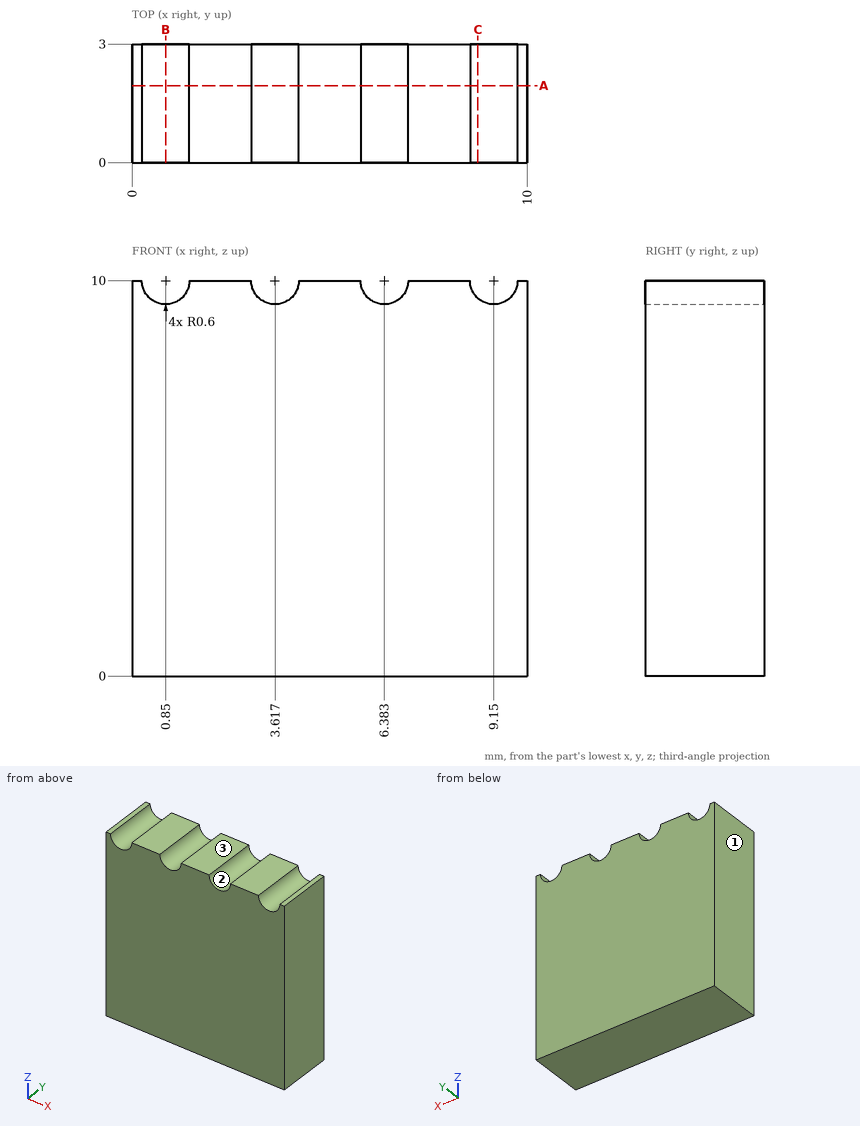
Part print with two shaded views. Sizes in mm from the minimum x, y, z corner. Round coordinates to 2 decimals unless told otherwise and drop trailing zeros. Order: outer loops, then holes, each group sorted by start corner. A loop starts at its lowest first (then second) coordinate and runs counter-clockwise, first axis right, second up. Notation, with made-up numbers: (86, 83) - (137, 83) arc R7 cw to (137, 90) - close; hole circle Ø7 at (22, 86). An arc over 180 degrees is marked (long way). Answer as CSV lines item,"result". Start each with the question number.
1. Saw through at B-B, the plane x = 0.85. Write the cut outline in (y, z).
2. Saw through at A-A, the plane y = 1.95. Write the cut outline in (x, z).
3. Saw through at C-C, the plane x = 8.75. Write the cut outline in (y, z).
4. Drill centre lines: L1, parallel to Z at x = 9.25, y = 1.7; L2, parallel to Z at x = 6, y = 1.6. Where is each one in solid material? Low to high. Write a range as [from, to].
5. Pull direction X, two halves, no side cores. Call the marked faces 1, 2 and 3: +X half, -X half, draft (parallel to the pull), parting line (faces both ways), or undercut.
Model answer:
1,outline,"(0, 0) - (3, 0) - (3, 9.4) - (0, 9.4) - close"
2,outline,"(0, 0) - (10, 0) - (10, 10) - (9.75, 10) arc R0.6 cw to (8.55, 10) - (6.98, 10) arc R0.6 cw to (5.78, 10) - (4.22, 10) arc R0.6 cw to (3.02, 10) - (1.45, 10) arc R0.6 cw to (0.25, 10) - (0, 10) - close"
3,outline,"(0, 0) - (3, 0) - (3, 9.55) - (0, 9.55) - close"
4,L1,"z = [0, 9.41]"
4,L2,"z = [0, 9.54]"
5,face 1,"-X half"
5,face 2,"undercut"
5,face 3,"draft"
